Part model, mm, in its own coordinate system. Face numbers are marked on the shaded views. A direction names the side the tool comes from. Round coordinates to 2 decimals unless told otherwise and drop trailing zeros. Loops run counter-clockwise (first coordinate to the right, second up) from the corner with the lowest first, then second, coordinate; pieces in that order, holes last. Notation, with made-up numbers: (64, 16.25) - (92, 16.25) arc R22 ccw to (92, 46.25) - close; hole circle Ø7 at (-9.5, -24.75). An arc over 180 degrees is marked (long way). Put each result on its own line as item: value.
from build123d import *

# Parameters (mm, degrees)
F1_DEPTH      = 12.7
F2_R          = 3.25
F3_DEPTH      = 24.131
F4_W          = 6.5
F4_H          = 6.5
F5_DEPTH      = 7.62
F6_W          = 70.85
F6_H          = 12.7
F7_DEPTH      = 19.05
F9_DEPTH      = 6.35
F10_W         = 14
F10_H         = 12.7
F11_DEPTH     = 7.62
F12_R         = 5
F13_R         = 3.025
F14_DEPTH     = 24.131
F15_R         = 5
F16_DEPTH     = 24.131
F17_R         = 5
F19_DEPTH     = 4
F20_T1_DEPTH  = 12.7
F20_T6_DEPTH  = 12.7
F20_T12_DEPTH = 12.7
F20_T18_DEPTH = 12.7
F20_T21_DEPTH = 31.0012701892
F22_DEPTH     = 12


# Not quite as in the source:
# - a fillet or chamfer that OpenCascade refuses, or shapes differently, is made with other operations: its cross-section is extruded or revolved along the edge and cut away or added


with BuildPart() as f1:
    # F0 (on Top) → F1 (new body, symmetric)
    with BuildSketch(Plane.XY):
        Polygon((11.43, 8.001), (11.43, -9.779), (4.826, -9.779), (-7.366, -9.779), (-11.43, -9.779), (-11.43, 8.001), (-17.78, 8.001), (-17.78, -16.129), (17.78, -16.129), (17.78, 8.001), align=None)
    extrude(amount=F1_DEPTH, both=True)

    # F2 (on face) → F3 (cut, through all)
    with BuildSketch(Plane.XZ.offset(16.129)):
        Circle(F2_R)
    extrude(amount=-F3_DEPTH, mode=Mode.SUBTRACT)

    # F4 (on face) → F5 (cut)
    with BuildSketch(Plane.XZ.offset(16.129)):
        Rectangle(F4_W, F4_H)
    extrude(amount=-F5_DEPTH, mode=Mode.SUBTRACT)

    # F6 (on face) → F7 (join)
    with BuildSketch(Plane.XY.offset(12.7)):
        with Locations((53.205, -9.779)):
            Rectangle(F6_W, F6_H)
    extrude(amount=-F7_DEPTH)

    # F8 (on face) → F9 (join)
    with BuildSketch(Plane.XZ.offset(16.129)):
        Polygon((17.78, -6.35), (17.78, -12.7), (43.18, -6.35), align=None)
    extrude(amount=-F9_DEPTH)

    # F10 (on face) → F11 (join)
    with BuildSketch(Plane.XY.offset(12.7)):
        with Locations((19.43, -9.779)):
            Rectangle(F10_W, F10_H)
        with Locations((75.43, -9.779)):
            Rectangle(F10_W, F10_H)
    extrude(amount=F11_DEPTH)

    # F12
    f12_edges = [f1.edges().sort_by_distance(p)[0] for p in [
        (26.43, -9.779, 20.32),
        (12.43, -9.779, 20.32),
        (68.43, -9.779, 20.32),
        (82.43, -9.779, 20.32),
    ]]
    fillet(f12_edges, radius=F12_R)

    # F13 (on face) → F14 (cut, through all)
    with BuildSketch(Plane.XZ.offset(16.129)):
        with Locations((19.43, 12.7)):
            Circle(F13_R)
        with Locations((75.43, 12.7)):
            Circle(F13_R)
    extrude(amount=-F14_DEPTH, mode=Mode.SUBTRACT)

    # F15 (on face) → F16 (cut, through all)
    with BuildSketch(Plane.XZ.offset(16.129)):
        with Locations((47.43, 12.7)):
            Circle(F15_R)
    extrude(amount=-F16_DEPTH, mode=Mode.SUBTRACT)

    # F17
    f17_edges = [f1.edges().sort_by_distance(p)[0] for p in [
        (42.43, -9.779, 12.7),
    ]]
    fillet(f17_edges, radius=F17_R)

    # F18 (on face) → F19 (cut)
    with BuildSketch(Plane(origin=(0, -3.429, 0), x_dir=(-1, 0, 0), z_dir=(0, 1, 0))):
        Polygon((-69.6564973081, 12.7), (-72.5432486541, 17.7), (-78.3167513459, 17.7), (-81.2035026919, 12.7), (-78.3167513459, 7.7), (-72.5432486541, 7.7), align=None)
        Polygon((-25.2035026919, 12.7), (-22.3167513459, 7.7), (-16.5432486541, 7.7), (-13.6564973081, 12.7), (-16.5432486541, 17.7), (-22.3167513459, 17.7), align=None)
    extrude(amount=-F19_DEPTH, mode=Mode.SUBTRACT)

    # F20: fillet of radius 5 on 5 edges, made by hand

    # F20_s2 → F20_t1 (join)
    with BuildSketch(Plane.XZ.offset(3.429)):
        with BuildLine():
            ThreePointArc((82.2863257716, 16.51), (84.0563916708, 13.7661723474), (87.1426515432, 12.7))
            Line((87.1426515432, 12.7), (87.1426515432, 12.2))
            Line((87.1426515432, 12.2), (82.43, 12.2))
            Line((82.43, 12.2), (81.93, 12.7))
            ThreePointArc((81.93, 12.7), (81.93, 15.32), (81.8006931944, 16.391))
            Line((81.8006931944, 16.391), (82.2863257716, 16.51))
        make_face()
        with BuildLine():
            ThreePointArc((63.7173484568, 12.7), (66.8036083292, 13.7661723474), (68.5736742284, 16.51))
            Line((68.5736742284, 16.51), (69.0593068056, 16.391))
            ThreePointArc((69.0593068056, 16.391), (68.93, 15.32), (68.93, 12.7))
            Line((68.93, 12.7), (68.43, 12.2))
            Line((68.43, 12.2), (63.7173484568, 12.2))
            Line((63.7173484568, 12.2), (63.7173484568, 12.7))
        make_face()
        with BuildLine():
            ThreePointArc((31.1426515432, 12.7), (28.0563916708, 13.7661723474), (26.2863257716, 16.51))
            Line((26.2863257716, 16.51), (25.8006931944, 16.391))
            ThreePointArc((25.8006931944, 16.391), (25.93, 15.32), (25.93, 12.7))
            Line((25.93, 12.7), (26.43, 12.2))
            Line((26.43, 12.2), (31.1426515432, 12.2))
            Line((31.1426515432, 12.2), (31.1426515432, 12.7))
        make_face()
    extrude(amount=F20_T1_DEPTH)


with BuildPart() as f20_tool4:
    # F20_s5 → F20_t6 (new body)
    with BuildSketch(Plane.XZ.offset(3.429)):
        with BuildLine():
            ThreePointArc((12.5736742284, 16.51), (10.8036083292, 13.7661723474), (7.7173484568, 12.7))
            Line((7.7173484568, 12.7), (7.7173484568, 12.2))
            Line((7.7173484568, 12.2), (12.43, 12.2))
            Line((12.43, 12.2), (12.93, 12.7))
            ThreePointArc((12.93, 12.7), (12.93, 15.32), (13.0593068056, 16.391))
            Line((13.0593068056, 16.391), (12.5736742284, 16.51))
        make_face()
    extrude(amount=F20_T6_DEPTH)

    split(bisect_by=Plane.XZ.offset(9.779), keep=Keep.BOTTOM)

    split(bisect_by=Plane.YZ.offset(11.43), keep=Keep.TOP)


with BuildPart() as f1_1:
    add(f1.part)

    # F20_t3: union F20_tool4
    add(f20_tool4.part)


with BuildPart() as f20_tool10:
    # F20_s11 → F20_t12 (new body)
    with BuildSketch(Plane.XZ.offset(3.429)):
        with BuildLine():
            ThreePointArc((12.5736742284, 16.51), (10.8036083292, 13.7661723474), (7.7173484568, 12.7))
            Line((7.7173484568, 12.7), (7.7173484568, 12.2))
            Line((7.7173484568, 12.2), (12.43, 12.2))
            Line((12.43, 12.2), (12.93, 12.7))
            ThreePointArc((12.93, 12.7), (12.93, 15.32), (13.0593068056, 16.391))
            Line((13.0593068056, 16.391), (12.5736742284, 16.51))
        make_face()
    extrude(amount=F20_T12_DEPTH)

    split(bisect_by=Plane.XZ.offset(9.779), keep=Keep.TOP)

    split(bisect_by=Plane.YZ.offset(11.43), keep=Keep.TOP)


with BuildPart() as f1_2:
    add(f1_1.part)

    # F20_t9: union F20_tool10
    add(f20_tool10.part)


with BuildPart() as f20_tool16:
    # F20_s17 → F20_t18 (new body)
    with BuildSketch(Plane.XZ.offset(3.429)):
        with BuildLine():
            ThreePointArc((12.5736742284, 16.51), (10.8036083292, 13.7661723474), (7.7173484568, 12.7))
            Line((7.7173484568, 12.7), (7.7173484568, 12.2))
            Line((7.7173484568, 12.2), (12.43, 12.2))
            Line((12.43, 12.2), (12.93, 12.7))
            ThreePointArc((12.93, 12.7), (12.93, 15.32), (13.0593068056, 16.391))
            Line((13.0593068056, 16.391), (12.5736742284, 16.51))
        make_face()
    extrude(amount=F20_T18_DEPTH)

    split(bisect_by=Plane.XZ.offset(9.779), keep=Keep.TOP)

    split(bisect_by=Plane.YZ.offset(11.43), keep=Keep.BOTTOM)


with BuildPart() as f1_3:
    add(f1_2.part)

    # F20_t15: union F20_tool16
    add(f20_tool16.part)

    # F20_s22 → F20_t21 (cut)
    with BuildSketch(Plane.XZ.offset(-5.7216350946)):
        with BuildLine():
            ThreePointArc((51.7601270189, 10.2), (53.5902540378, 12.0301270189), (56.0902540378, 12.7))
            Line((56.0902540378, 12.7), (52.43, 12.7))
            ThreePointArc((52.43, 12.7), (52.2596291314, 11.4059047745), (51.7601270189, 10.2))
        make_face()
    extrude(amount=F20_T21_DEPTH, mode=Mode.SUBTRACT)

    # F21 (on face) → F22 (cut)
    with BuildSketch(Plane(origin=(0, 8.001, 0), x_dir=(-1, 0, 0), z_dir=(0, 1, 0))):
        Polygon((-22.3456188594, 7.65), (-16.5143811406, 7.65), (-13.5987622812, 12.7), (-16.5143811406, 17.75), (-22.3456188594, 17.75), (-25.2612377188, 12.7), align=None)
    extrude(amount=-F22_DEPTH, mode=Mode.SUBTRACT)


solid = f1_3.part
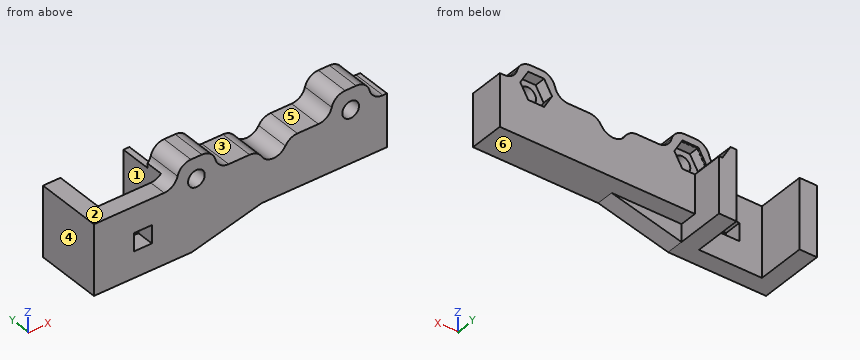
1. Band-saw the part on C-C (z = 1.5). List the corners of the cut face in (x, y), plus the area to 3 significant figures.
A:
outline: (-17.78, -16.13) - (-3.25, -16.13) - (-3.25, -9.78) - (-11.43, -9.78) - (-11.43, 8) - (-17.78, 8) - close; (3.25, -16.13) - (88.63, -16.13) - (88.63, -3.43) - (17.78, -3.43) - (17.78, 8) - (11.43, 8) - (11.43, -9.78) - (3.25, -9.78) - close
area: 1,310 mm²
2. Band-saw the part on D-D (y = -1.5). List the corners of the cut face in (x, z), plus the area to 3 significant figures.
A:
outline: (-17.78, -12.7) - (-11.43, -12.7) - (-11.43, 12.7) - (-17.78, 12.7) - close; (11.43, -12.7) - (17.78, -12.7) - (17.78, 7.65) - (16.51, 7.65) - (13.6, 12.7) - (11.43, 12.7) - close
area: 309 mm²
3. Band-saw the part on B-B (y = -8.5). List the corners of the cut face in (x, z) (3 decimals).
A:
outline: (-17.78, -12.7) - (-11.43, -12.7) - (-11.43, 12.7) - (-17.78, 12.7) - close; (11.43, -12.7) - (17.78, -12.7) - (17.78, -6.35) - (88.63, -6.35) - (88.63, 12.7) - (87.143, 12.7) arc R5 cw to (82.286, 16.51) arc R5 ccw to (77.43, 20.32) - (73.43, 20.32) arc R5 ccw to (68.574, 16.51) arc R5 cw to (63.717, 12.7) - (56.09, 12.7) arc R5 ccw to (51.76, 10.2) arc R5 cw to (43.1, 10.2) arc R5 ccw to (38.77, 12.7) - (31.143, 12.7) arc R5 cw to (26.286, 16.51) arc R5 ccw to (21.43, 20.32) - (17.43, 20.32) arc R5 ccw to (12.574, 16.51) arc R5 cw to (11.43, 14.351) - close; hole circle Ø6.05 at (19.43, 12.7); hole circle Ø6.05 at (75.43, 12.7)
4. Two-plate mould, pull along X, no slides. Class the marked faces 4, 5 and 6: pulls with the +X half, pulls with the -X half, needs draft (parallel to the pull), parting line crosses it, or undercut.
A:
face 4: pulls with the -X half
face 5: undercut
face 6: needs draft
5. Pin check, flat tips, straight feed: P1, Ø6, axis at x = -1.5, z = 9.5, coming from the +Y side; P2, Ø6, axis at x = 62, y = -7, coming from the +Z side; P3, Ø3, axis at x = 22, z = 10.5, coming from the +Y side; P4, Ø5, axis at x = 75.43, z = 12.7, coming from the +Y side. Stop position of each tip, or through.
A:
P1: stops at y = -9.78
P2: stops at z = 12.87
P3: stops at y = -7.43
P4: passes through
6. Tool access for the marked faces 1, 2 and 3: list every direction of +Z, -Z, +X, -X, +Y, -Y with a clear straight run to the whole face (end or side of a thin tool).
A:
face 1: +Z, -Z, +Y
face 2: +Z, -X, +Y, -Y
face 3: +Z, +Y, -Y
7. Band-saw the part on A-A (x = 75.43). List the corners of the cut face in (y, z) (3 decimals), plus the area to 3 significant figures.
A:
outline: (-16.129, -6.35) - (-3.429, -6.35) - (-3.429, 7.7) - (-7.429, 7.7) - (-7.429, 9.675) - (-16.129, 9.675) - close; (-16.129, 15.725) - (-7.429, 15.725) - (-7.429, 17.7) - (-3.429, 17.7) - (-3.429, 20.32) - (-16.129, 20.32) - close
area: 246 mm²
8. Probe line 1 along X through (y, z) = (-3.75, -4); line 2 along Z through (x, y) = (2, -14); line 3 along Z through (x, y) = (75.43, -10) (3 decimals). List the from-to ranges inside material, lowest first. Write a range as [from, to].
A:
line 1: x = [-17.78, -11.43], [11.43, 88.63]
line 2: z = [-12.7, -3.25], [3.25, 12.7]
line 3: z = [-6.35, 9.675], [15.725, 20.32]
